Work out the finished part from the listing and answer in its coordinate system (mm). Face numbers are marked on the shaded views. A direction names the side the tool comes from. Round coordinates to 2 decimals unless told otherwise and drop trailing zeros. Write each loop counter-clockwise with the first axis right and the second up, starting at its lowest first coordinate (ties: lowest second). Pieces come first, ordered by that corner, then holes. Notation, with made-up numbers: (-28, 44.5) -> (11, 44.5) arc R16 cw to (11, 55.5) -> close; hole circle Ø1 at (34.25, 75.25). An arc over 180 degrees is marked (long way). One line per item, written item: value.
```python
from build123d import *

# Parameters (mm, degrees)
SKETCH2_R               = 2.4892
BOSS_EXTRUDE1_DEPTH     = 3.175
SKETCH3_R               = 2.4892
CUT_EXTRUDE1_DEPTH      = 143.74264703
EDGE_FLANGE1_DEPTH      = 130.175
EDGE_FLANGE1_BEND_DEPTH = 130.175
CUT_EXTRUDE2_DEPTH      = 275.581526204
EDGE_FLANGE2_DEPTH      = 25.4
EDGE_FLANGE2_BEND_DEPTH = 25.4
CUT_EXTRUDE3_REACH      = 159.273
SKETCH22_R              = 2.4892
FILLET2_R               = 6.35
SKETCH23_R              = 2.4892
CUT_EXTRUDE4_DEPTH      = 276.337091157
CUT_EXTRUDE5_REACH      = 277.337
SKETCH24_R              = 1.42494


# Sheet-metal steps are written as plain solids
with BuildPart() as part:
    # Sketch2 → Boss-Extrude1 (new body)
    with BuildSketch(Plane(origin=(0, 0, 0), x_dir=(1, 0, 0), z_dir=(0, 1, 0))):
        Polygon((-127, 65.0875), (-127, -65.0875), (127, -65.0875), (127, 65.0875), (101.6, 65.0875), (101.6, -39.624), (-101.6, -39.624), (-101.6, 65.0875), align=None)
        with Locations(Location((-114.3, 26.9875, 0), (0, 0, 270))):
            Circle(SKETCH2_R, mode=Mode.SUBTRACT)
        with Locations(Location((-114.3, 39.6875, 0), (0, 0, 270))):
            Circle(SKETCH2_R, mode=Mode.SUBTRACT)
        with Locations(Location((-114.3, 52.3875, 0), (0, 0, 270))):
            Circle(SKETCH2_R, mode=Mode.SUBTRACT)
        with Locations(Location((114.3, 26.9875, 0), (0, 0, 270))):
            Circle(SKETCH2_R, mode=Mode.SUBTRACT)
        with Locations(Location((114.3, 39.6875, 0), (0, 0, 270))):
            Circle(SKETCH2_R, mode=Mode.SUBTRACT)
        with Locations(Location((114.3, 52.3875, 0), (0, 0, 270))):
            Circle(SKETCH2_R, mode=Mode.SUBTRACT)
    extrude(amount=BOSS_EXTRUDE1_DEPTH)

    # Sketch3 → Cut-Extrude1 (cut, through all)
    with BuildSketch(Plane(origin=(0, 3.175, 0), x_dir=(1, 0, 0), z_dir=(0, 1, 0))):
        with Locations(Location((-102.87, -55.5625, 0), (0, 0, 270))):
            Circle(SKETCH3_R)
        with Locations(Location((-80.01, -55.5625, 0), (0, 0, 270))):
            Circle(SKETCH3_R)
        with Locations(Location((-114.3, -55.5625, 0), (0, 0, 270))):
            Circle(SKETCH3_R)
        with Locations(Location((-57.15, -55.5625, 0), (0, 0, 270))):
            Circle(SKETCH3_R)
        with Locations(Location((114.3, -55.5625, 0), (0, 0, 270))):
            Circle(SKETCH3_R)
        with Locations(Location((-34.29, -55.5625, 0), (0, 0, 270))):
            Circle(SKETCH3_R)
        with Locations(Location((-11.43, -55.5625, 0), (0, 0, 270))):
            Circle(SKETCH3_R)
        with Locations(Location((11.43, -55.5625, 0), (0, 0, 270))):
            Circle(SKETCH3_R)
        with Locations(Location((34.29, -55.5625, 0), (0, 0, 270))):
            Circle(SKETCH3_R)
        with Locations(Location((57.15, -55.5625, 0), (0, 0, 270))):
            Circle(SKETCH3_R)
        with Locations(Location((80.01, -55.5625, 0), (0, 0, 270))):
            Circle(SKETCH3_R)
        with Locations(Location((102.87, -55.5625, 0), (0, 0, 270))):
            Circle(SKETCH3_R)
    extrude(amount=-CUT_EXTRUDE1_DEPTH, mode=Mode.SUBTRACT)

    # Edge-Flange1 section (across the edge) → Edge-Flange1 (add)
    with BuildSketch(Plane(origin=(127.762, 0, -65.0875), x_dir=(-1, 0, 0), z_dir=(0, 0, 1))):
        with BuildLine():
            Line((-3.175, 0.762), (-3.175, 50.8))
            Line((-3.175, 50.8), (0, 50.8))
            Line((0, 50.8), (0, 0.762))
            ThreePointArc((0, 0.762), (0.223184633, 0.223184633), (0.762, 0))
            Line((0.762, 0), (0.762, -3.175))
            ThreePointArc((0.762, -3.175), (-2.021879398, -2.021879398), (-3.175, 0.762))
        make_face()
    extrude(amount=EDGE_FLANGE1_DEPTH)

    # Edge-Flange1 section 2 (across the edge) → Edge-Flange1 bend (add)
    with BuildSketch(Plane(origin=(-127.762, 0, 65.0875), x_dir=(1, 0, 0), z_dir=(0, 0, -1))):
        with BuildLine():
            Line((-3.175, 0.762), (-3.175, 50.8))
            Line((-3.175, 50.8), (0, 50.8))
            Line((0, 50.8), (0, 0.762))
            ThreePointArc((0, 0.762), (0.223184633, 0.223184633), (0.762, 0))
            Line((0.762, 0), (0.762, -3.175))
            ThreePointArc((0.762, -3.175), (-2.021879398, -2.021879398), (-3.175, 0.762))
        make_face()
    extrude(amount=EDGE_FLANGE1_BEND_DEPTH)

    # Sketch15 → Cut-Extrude2 (cut, through all)
    with BuildSketch(Plane(origin=(130.937, 0, 0), x_dir=(0, 0, -1), z_dir=(1, 0, 0))):
        with BuildLine():
            Line((-39.6875, -47.228125), (-39.6875, -50.8))
            Line((-39.6875, -50.8), (-37.30625, -50.8))
            Line((-37.30625, -50.8), (-37.30625, -47.228125))
            ThreePointArc((-37.30625, -47.228125), (-37.654975989, -46.386225989), (-38.496875, -46.0375))
            ThreePointArc((-38.496875, -46.0375), (-39.338774011, -46.386225989), (-39.6875, -47.228125))
        make_face()
    extrude(amount=-CUT_EXTRUDE2_DEPTH, mode=Mode.SUBTRACT)

    # Edge-Flange2 section (across the edge) → Edge-Flange2 (add)
    with BuildSketch(Plane(origin=(127.762, -51.562, 39.6875), x_dir=(0, 1, 0), z_dir=(0, 0, 1))):
        with BuildLine():
            Line((-3.175, 0.762), (-3.175, 31.75))
            Line((-3.175, 31.75), (0, 31.75))
            Line((0, 31.75), (0, 0.762))
            ThreePointArc((0, 0.762), (0.223184633, 0.223184633), (0.762, 0))
            Line((0.762, 0), (0.762, -3.175))
            ThreePointArc((0.762, -3.175), (-2.021879398, -2.021879398), (-3.175, 0.762))
        make_face()
    extrude(amount=EDGE_FLANGE2_DEPTH)

    # Edge-Flange2 section 2 (across the edge) → Edge-Flange2 bend (add)
    with BuildSketch(Plane(origin=(-127.762, -51.562, 65.0875), x_dir=(0, 1, 0), z_dir=(0, 0, -1))):
        with BuildLine():
            Line((-3.175, 0.762), (-3.175, 31.75))
            Line((-3.175, 31.75), (0, 31.75))
            Line((0, 31.75), (0, 0.762))
            ThreePointArc((0, 0.762), (0.223184633, 0.223184633), (0.762, 0))
            Line((0.762, 0), (0.762, -3.175))
            ThreePointArc((0.762, -3.175), (-2.021879398, -2.021879398), (-3.175, 0.762))
        make_face()
    extrude(amount=EDGE_FLANGE2_BEND_DEPTH)

    # Sketch22 → Cut-Extrude3 (cut, up to next)
    with BuildSketch(Plane.XZ.offset(54.737), mode=Mode.PRIVATE) as cut_extrude3_sk1:
        with Locations(Location((-102.87, 55.5625, 0), (0, 0, 90))):
            Circle(SKETCH22_R)
    cut_extrude3_tool1 = extrude(cut_extrude3_sk1.sketch, amount=-CUT_EXTRUDE3_REACH, mode=Mode.PRIVATE) & part.part
    # Sketch22 → Cut-Extrude3 (cut, up to next)
    with BuildSketch(Plane.XZ.offset(54.737), mode=Mode.PRIVATE) as cut_extrude3_sk2:
        with Locations(Location((-114.3, 55.5625, 0), (0, 0, 90))):
            Circle(SKETCH22_R)
    cut_extrude3_tool2 = extrude(cut_extrude3_sk2.sketch, amount=-CUT_EXTRUDE3_REACH, mode=Mode.PRIVATE) & part.part
    # Sketch22 → Cut-Extrude3 (cut, up to next)
    with BuildSketch(Plane.XZ.offset(54.737), mode=Mode.PRIVATE) as cut_extrude3_sk3:
        with Locations(Location((102.87, 55.5625, 0), (0, 0, 90))):
            Circle(SKETCH22_R)
    cut_extrude3_tool3 = extrude(cut_extrude3_sk3.sketch, amount=-CUT_EXTRUDE3_REACH, mode=Mode.PRIVATE) & part.part
    # Sketch22 → Cut-Extrude3 (cut, up to next)
    with BuildSketch(Plane.XZ.offset(54.737), mode=Mode.PRIVATE) as cut_extrude3_sk4:
        with Locations(Location((114.3, 55.5625, 0), (0, 0, 90))):
            Circle(SKETCH22_R)
    cut_extrude3_tool4 = extrude(cut_extrude3_sk4.sketch, amount=-CUT_EXTRUDE3_REACH, mode=Mode.PRIVATE) & part.part
    add(cut_extrude3_tool1.solids().sort_by_distance((-102.87, -54.737, 55.5625))[0], mode=Mode.SUBTRACT)
    add(cut_extrude3_tool2.solids().sort_by_distance((-114.3, -54.737, 55.5625))[0], mode=Mode.SUBTRACT)
    add(cut_extrude3_tool3.solids().sort_by_distance((102.87, -54.737, 55.5625))[0], mode=Mode.SUBTRACT)
    add(cut_extrude3_tool4.solids().sort_by_distance((114.3, -54.737, 55.5625))[0], mode=Mode.SUBTRACT)

    # Fillet2
    fillet2_edges = [part.edges().sort_by_distance(p)[0] for p in [
        (96.012, -53.1495, 65.0875),
        (96.012, -53.1495, 39.6875),
        (129.3495, -50.8, -65.0875),
        (101.6, 1.5875, -65.0875),
        (101.6, 1.5875, 39.624),
        (-101.6, 1.5875, 39.624),
        (-101.6, 1.5875, -65.0875),
        (-129.3495, -50.8, -65.0875),
        (-96.012, -53.1495, 65.0875),
        (-96.012, -53.1495, 39.6875),
        (129.3495, -50.8, 37.30625),
        (-129.3495, -50.8, 37.30625),
    ]]
    fillet(fillet2_edges, radius=FILLET2_R)

    # Sketch23 → Cut-Extrude4 (cut, through all)
    with BuildSketch(Plane(origin=(130.937, 0, 0), x_dir=(0, 0, -1), z_dir=(1, 0, 0))):
        with Locations(Location((52.3875, -12.7, 0), (0, 0, 90))):
            Circle(SKETCH23_R)
        with Locations(Location((39.6875, -12.7, 0), (0, 0, 90))):
            Circle(SKETCH23_R)
        with Locations(Location((26.9875, -12.7, 0), (0, 0, 90))):
            Circle(SKETCH23_R)
    extrude(amount=-CUT_EXTRUDE4_DEPTH, mode=Mode.SUBTRACT)

    # Sketch24 → Cut-Extrude5 (cut, up to next)
    with BuildSketch(Plane(origin=(130.937, 0, 0), x_dir=(0, 0, -1), z_dir=(1, 0, 0)), mode=Mode.PRIVATE) as cut_extrude5_sk1:
        with Locations(Location((-23.8125, -38.1, 0), (0, 0, 90))):
            Circle(SKETCH24_R)
    cut_extrude5_tool1 = extrude(cut_extrude5_sk1.sketch, amount=-CUT_EXTRUDE5_REACH, mode=Mode.PRIVATE) & part.part
    # Sketch24 → Cut-Extrude5 (cut, up to next)
    with BuildSketch(Plane(origin=(130.937, 0, 0), x_dir=(0, 0, -1), z_dir=(1, 0, 0)), mode=Mode.PRIVATE) as cut_extrude5_sk2:
        with Locations(Location((-23.8125, -30.099999998, 0), (0, 0, 90))):
            Circle(SKETCH24_R)
    cut_extrude5_tool2 = extrude(cut_extrude5_sk2.sketch, amount=-CUT_EXTRUDE5_REACH, mode=Mode.PRIVATE) & part.part
    add(cut_extrude5_tool1.solids().sort_by_distance((130.937, -38.1, 23.8125))[0], mode=Mode.SUBTRACT)
    add(cut_extrude5_tool2.solids().sort_by_distance((130.937, -30.1, 23.8125))[0], mode=Mode.SUBTRACT)


solid = part.part
```
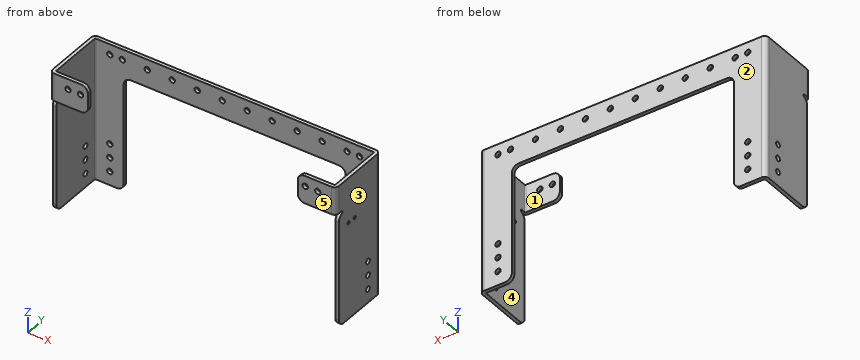
(1) A tool of negligible diameter and unlimited length cuts with its end or side. For the marked faces 1 and 2, from which of +Z, -Z, +X, -X, +Y, -Y can it reach the whole face along a straight path? Write none if from no direction.
Reported:
face 1: +Z, -Z
face 2: +Z, -Z, +X, -X, +Y
(2) Find section B-B on y = -22. Give the vertices of the cut face in (x, z).
Reported:
outline: (-130.94, -65.09) -> (-127.76, -65.09) -> (-127.76, 65.09) -> (-130.94, 65.09) -> close; (127.76, -65.09) -> (130.94, -65.09) -> (130.94, 65.09) -> (127.76, 65.09) -> close
(3) For a pull along Y with two mould halves and no side action, classify the marked faces 3, 4 and 5 as pulls with the +Y half, pulls with the -Y half, needs draft (parallel to the pull), parting line crosses it, or undercut.
Reported:
face 3: needs draft
face 4: undercut
face 5: pulls with the -Y half
(4) Flat-ended cylindrical pins translate along their axes: pin 1 Ø4.5 at (x, z) = (114.3, 55.56) entering from -Y; pin 2 Ø3.5 at (y, z) = (1.5, -33.5) entering from -X; pin 3 Ø3.5 at (x, y) = (-1.5, 1) entering from -Z; pin 4 Ø8.5 at (x, y) = (121.5, -52) entering from -Z. Find the tip coordinate at first contact, or state that the pin passes through.
Reported:
pin 1: passes through
pin 2: stops at x = -130.9
pin 3: stops at z = 39.62
pin 4: stops at z = 39.69
(5) Find section C-C on z = -14. Give the vertices of the cut face in (x, y) (3 decimals), plus the area to 3 significant figures.
Reported:
outline: (-130.937, -50.8) -> (-127.762, -50.8) -> (-127.762, -0.762) arc R0.762 cw to (-127, 0) -> (-101.6, 0) -> (-101.6, 3.175) -> (-127, 3.175) arc R3.937 ccw to (-130.937, -0.762) -> close; (101.6, 0) -> (127, 0) arc R0.762 cw to (127.762, -0.762) -> (127.762, -50.8) -> (130.937, -50.8) -> (130.937, -0.762) arc R3.937 ccw to (127, 3.175) -> (101.6, 3.175) -> close
area: 502 mm2
(6) Find section D-D on x = 46.5. Give the vertices of the cut face in (y, z) (1 decimal), plus the area to 3 significant figures.
Reported:
outline: (0, 39.6) -> (3.2, 39.6) -> (3.2, 65.1) -> (0, 65.1) -> close
area: 80.8 mm2
(7) Consider probe 1 along X at (y, z) = (-24, 9.5); probe 2 along Z at (x, y) = (128, -12); probe 3 along Y at (x, z) = (105, 32) (3 decimals). Determine where each line is inside the solid, lowest interval first.
Reported:
probe 1: x = -130.94 to -127.76, 127.76 to 130.94
probe 2: z = -65.09 to -54.78, -50 to -42.08, -37.3 to -29.38, -24.6 to 65.09
probe 3: y = 0 to 3.175
(8) Find section A-A on x = -34.29. Give the vertices of the cut face in (y, z) (1 decimal).
Reported:
outline: (0, 39.6) -> (3.2, 39.6) -> (3.2, 53.1) -> (0, 53.1) -> close; (0, 58.1) -> (3.2, 58.1) -> (3.2, 65.1) -> (0, 65.1) -> close
